Read the model definition and answer for the solid it produces. Units are mm, in the model's axes. Face numbers are marked on the shaded views. Coordinates: 2 decimals unless noted, no trailing zeros. Write each loop counter-clockwise with the first axis right and the second up, starting at its lowest first coordinate (ties: lowest second). Pieces come first, ordered by that corner, then holes. Notation, with made-up numbers: (1.5, 19) -> (35.5, 19) arc R18 ccw to (35.5, 26) -> close; hole circle Ø4 at (73.5, 39.5). An arc over 180 degrees is marked (long way). Answer in a Markdown table with one row per item. Add a question column.
Item 1: Given pin 1 Ø5 at (x, y) = (0, 0) entering from +Z; pin 2 Ø1.5 at (y, z) = (-3, 2.5) entering from +X, each flat-ended and moving along its own axis, determine where each tip first touches the part or whether it passes through.
Item 2: For a pull along X with two mould halves and no side action, classify the marked faces 1, 2 and 3 as +X half, -X half, draft (parallel to the pull), parting line (faces both ways), or undercut.
Item 3: Section A-A on z = 1 is taken. Write down the section's boundary in (x, y), then the cut area to 3 significant figures.
Item 4: Straight lines are drawn through the part: line 1 (Y direction, x = 0, z = 3.1); line 2 (Y direction, x = 2, z = 3.5); line 3 (X direction, y = -1, z = 3.75). For each, find the intervals that lie inside material, in ascending order. Write a range as from..to.
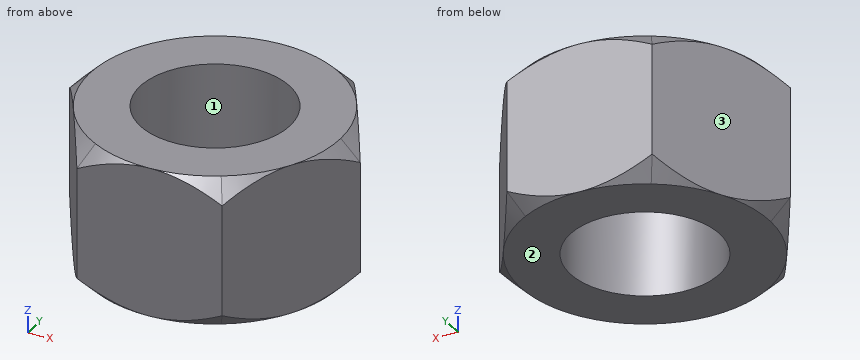
```python
from build123d import *

# Parameters (mm, degrees)
F0_R     = 3
F1_DEPTH = 6
F2_SIZE  = 0.7735
F3_DEPTH = 6.001


# Not quite as in the source:
# - a feature names something its author has since deleted; it is built from what else it names


with BuildPart() as f1:
    # F0 (on Top) → F1 (new body)
    with BuildSketch(Plane.XY):
        Polygon((2.8867513459, 5), (-2.8867513459, 5), (-5.7735026919, 0), (-2.8867513459, -5), (2.8867513459, -5), (5.7735026919, 0), align=None)
        Circle(F0_R, mode=Mode.SUBTRACT)
        with BuildLine():
            Line((-5.7735026919, 0), (-2.8867513459, 5))
            ThreePointArc((-2.8867513459, 5), (-5, 2.8867513459), (-5.7735026919, 0))
        make_face()
        with BuildLine():
            Line((-2.8867513459, -5), (-5.7735026919, 0))
            ThreePointArc((-5.7735026919, 0), (-5, -2.8867513459), (-2.8867513459, -5))
        make_face()
        with BuildLine():
            ThreePointArc((2.8867513459, -5), (5, -2.8867513459), (5.7735026919, 0))
            Line((5.7735026919, 0), (2.8867513459, -5))
        make_face()
        with BuildLine():
            ThreePointArc((5.7735026919, 0), (5, 2.8867513459), (2.8867513459, 5))
            Line((2.8867513459, 5), (5.7735026919, 0))
        make_face()
        with BuildLine():
            ThreePointArc((2.8867513459, 5), (0, 5.7735026919), (-2.8867513459, 5))
            Line((-2.8867513459, 5), (2.8867513459, 5))
        make_face()
        with BuildLine():
            Line((2.8867513459, -5), (-2.8867513459, -5))
            ThreePointArc((-2.8867513459, -5), (0, -5.7735026919), (2.8867513459, -5))
        make_face()
    extrude(amount=F1_DEPTH)

    # F2
    f2_edges = [f1.edges().sort_by_distance(p)[0] for p in [
        (2.886751, 5, 6),
        (2.886751, 5, 0),
    ]]
    chamfer(f2_edges, length=F2_SIZE)

    # F0 (on Top) → F3 (cut, through all)
    with BuildSketch(Plane.XY):
        with BuildLine():
            Line((-2.8867513459, -5), (-5.7735026919, 0))
            ThreePointArc((-5.7735026919, 0), (-5, -2.8867513459), (-2.8867513459, -5))
        make_face()
        with BuildLine():
            Line((-5.7735026919, 0), (-2.8867513459, 5))
            ThreePointArc((-2.8867513459, 5), (-5, 2.8867513459), (-5.7735026919, 0))
        make_face()
        with BuildLine():
            ThreePointArc((2.8867513459, 5), (0, 5.7735026919), (-2.8867513459, 5))
            Line((-2.8867513459, 5), (2.8867513459, 5))
        make_face()
        with BuildLine():
            ThreePointArc((5.7735026919, 0), (5, 2.8867513459), (2.8867513459, 5))
            Line((2.8867513459, 5), (5.7735026919, 0))
        make_face()
        with BuildLine():
            ThreePointArc((2.8867513459, -5), (5, -2.8867513459), (5.7735026919, 0))
            Line((5.7735026919, 0), (2.8867513459, -5))
        make_face()
        with BuildLine():
            Line((2.8867513459, -5), (-2.8867513459, -5))
            ThreePointArc((-2.8867513459, -5), (0, -5.7735026919), (2.8867513459, -5))
        make_face()
    extrude(amount=F3_DEPTH, mode=Mode.SUBTRACT)


solid = f1.part
```
Results below:
| question | item | result |
|---|---|---|
| 1 | pin 1 | passes through |
| 1 | pin 2 | stops at x = 4.47 |
| 2 | face 1 | undercut |
| 2 | face 2 | draft |
| 2 | face 3 | -X half |
| 3 | outline | (-5.77, 0) -> (-2.89, -5) -> (2.89, -5) -> (5.77, 0) -> (2.89, 5) -> (-2.89, 5) -> close; hole circle Ø6 at (0, 0) |
| 3 | area | 58.3 mm2 |
| 4 | line 1 | y = -5..-3, 3..5 |
| 4 | line 2 | y = -5..-2.24, 2.24..5 |
| 4 | line 3 | x = -5.2..-2.83, 2.83..5.2 |
